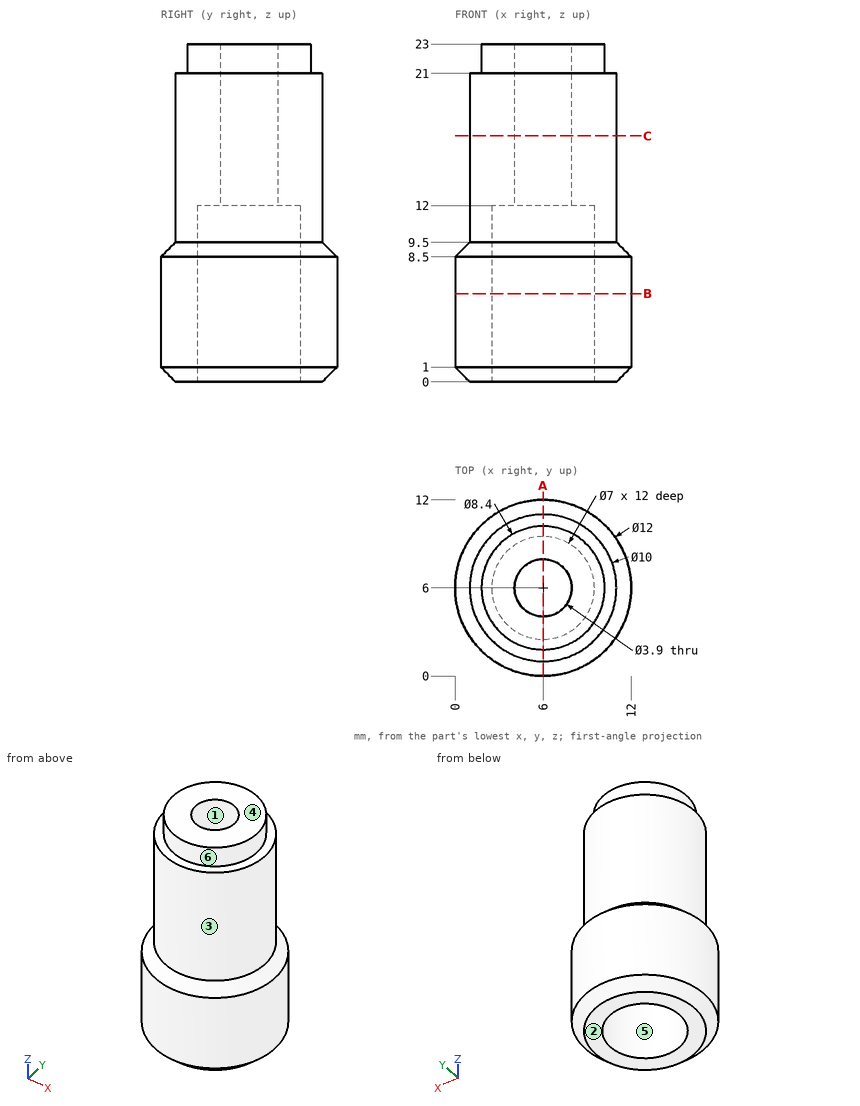
Job drawing, mm, ordinate dimensions from the low corner. One solid piece. A direction names the side the tool comes from. Give positions to 0.01 mm unless a question says otherwise; leave off trailing zeros. Order: outer loops, then holes, each group sorted by start corner. A loop starts at its lowest first (then second) coordinate and runs counter-clockwise, first axis right, second up. Notation, with made-up numbers: (30.5, 48) - (66.5, 48) arc R29 cw to (66.5, 73) - close; hole circle Ø8 at (57.5, 16). An arc over 180 degrees is marked (long way). Answer in a Markdown table with one row per item.
1. Tool access for the marked faces 4, 5 and 6: list every direction of +Z, -Z, +X, -X, +Y, -Y with a clear straight run to the whole face (end or side of a thin tool).
Data:
| item | result |
|---|---|
| face 4 | +Z, +X, -X, +Y, -Y |
| face 5 | -Z |
| face 6 | +Z |
2. Saw through at A-A, the plane x = 6. Give the cut face in (y, z), plus the area to 3 significant figures.
Data:
| item | result |
|---|---|
| outline | (0, 1) - (1, 0) - (2.5, 0) - (2.5, 12) - (4.05, 12) - (4.05, 23) - (1.8, 23) - (1.8, 21) - (1, 21) - (1, 9.5) - (0, 8.5) - close; (7.95, 12) - (9.5, 12) - (9.5, 0) - (11, 0) - (12, 1) - (12, 8.5) - (11, 9.5) - (11, 21) - (10.2, 21) - (10.2, 23) - (7.95, 23) - close |
| area | 117 mm² |
3. Saw through at C-C, the plane z = 16.75. Give the cut face in (x, y).
Data:
| item | result |
|---|---|
| outline | circle Ø10 at (6, 6); hole circle Ø3.9 at (6, 6) |
4. Pull direction Y, two halves, no side cores. Call the marked faces 1, 2 and 3: pulls with the +Y half, pulls with the -Y half, needs draft (parallel to the pull), parting line crosses it, or undercut.
Data:
| item | result |
|---|---|
| face 1 | undercut |
| face 2 | needs draft |
| face 3 | parting line crosses it |
5. Saw through at B-B, the plane z = 6. Give the cut face in (x, y).
Data:
| item | result |
|---|---|
| outline | circle Ø12 at (6, 6); hole circle Ø7 at (6, 6) |
6. Probe probe 1 along Y at (x, z) = (6, 18); probe 2 along Y at (x, z) = (6, 5.5); probe 3 along Z at (x, y) = (5, 3.5). List the from-to ranges inside material, lowest first. Write a range as [from, to].
Data:
| item | result |
|---|---|
| probe 1 | y = [1, 4.05], [7.95, 11] |
| probe 2 | y = [0, 2.5], [9.5, 12] |
| probe 3 | z = [12, 23] |
7. Flat gauge pins, fed straight in: pin 1 (3 mm diameter, centred on y = 3, z = 5, fed in from -X); pin 2 (1.5 mm diameter, centred on y = 10, z = 11, fed in from -X); pin 3 (6 mm diameter, centred on x = 6, z = 18, fed in from -Y). Where does each tip first touch, or does it go through?
Data:
| item | result |
|---|---|
| pin 1 | stops at x = 0.19 |
| pin 2 | stops at x = 2.2 |
| pin 3 | stops at y = 1 |
